The listing builds one solid part. Answer for the finished solid, in the listing's coordinates (mm). A direction names the side the tool comes from. Coordinates: 2 decimals unless noted, no trailing zeros. Order: outer loops, then holes, each group sorted by start corner. A loop starts at its lowest first (then second) coordinate and runs counter-clockwise, first axis right, second up.
from build123d import *

# Parameters (mm, degrees)
F0_R     = 47.826909
F0_R_2   = 27.35277
F1_DEPTH = 12.5
F2_R     = 35.491808
F2_R_2   = 27.557279
F3_DEPTH = 25
F4_R     = 47.701189
F4_R_2   = 35.254813
F5_DEPTH = 12.5
F6_R     = 48.078981
F6_R_2   = 35.711938
F7_DEPTH = 25
F8_R     = 47.890456
F8_R_2   = 35.598206
F9_DEPTH = 25


with BuildPart() as f1:
    # F0 (on Top) → F1 (new body, symmetric)
    with BuildSketch(Plane.XY):
        Circle(F0_R)
        Circle(F0_R_2, mode=Mode.SUBTRACT)
    extrude(amount=F1_DEPTH, both=True)

    # F2 (on Top) → F3 (join, symmetric)
    with BuildSketch(Plane.XY):
        Circle(F2_R)
        Circle(F2_R_2, mode=Mode.SUBTRACT)
    extrude(amount=F3_DEPTH, both=True)

    # F4 (on Top) → F5 (join, symmetric)
    with BuildSketch(Plane.XY):
        Circle(F4_R)
        Circle(F4_R_2, mode=Mode.SUBTRACT)
    extrude(amount=F5_DEPTH, both=True)

    # F6 (on Top) → F7 (cut)
    with BuildSketch(Plane.XY):
        Circle(F6_R)
        Circle(F6_R_2, mode=Mode.SUBTRACT)
    extrude(amount=-F7_DEPTH, mode=Mode.SUBTRACT)

    # F8 (on Top) → F9 (join)
    with BuildSketch(Plane.XY):
        Circle(F8_R)
        Circle(F8_R_2, mode=Mode.SUBTRACT)
    extrude(amount=F9_DEPTH)


solid = f1.part
1) A tool of negligible diameter and unlimited length cuts with its end or side. For faces 4 (the face through (26.285, 8.277, 18.662)), 5 (the face through (26.285, 8.277, -18.838)), 6 (the face through (0, 36, 25)), from which of +Z, -Z, +X, -X, +Y, -Y can it reach the whole face along a straight path? Write none if from no direction.
2) Determine the mould class of faces 1 (the face through (18.2, -20.9, 25)), 2 (the face through (34.06, 10.73, -6.16)), 3 (the face through (-21.71, -16.64, -0.18)) for opening direction Y: released by +Y, released by -Y, zero draft, split by the parting line, or undercut.
3) Section C-C (z = 4) is taken. Give the vertices of the cut face in (x, y), then the cut area to 3 significant figures.
4) Each of these flat-tipped pins is pushed along its axis until it touches: P1, Ø6, axis at x = -28, z = -7.5, coming from the +Y side; P2, Ø5, axis at x = -30, z = -17, coming from the +Y side; P3, Ø2, axis at x = 29, z = -15.5, coming from the +Y side. Where does it stop, or does it pass through?
5) Consider L1, parallel to Y at x = 0, z = -21.5; L2, parallel to Y at x = 0, z = 7.5; L3, parallel to Z at x = 6.5, y = 40. Determine where each line is inside the solid, lowest interval first.
6) Section D-D (y = -34) is taken. Give the vertices of the cut face in (x, z), then the cut area to 3 significant figures.
Filled sheet:
1. face 4: +Z
1. face 5: -Z
1. face 6: +Z, +X, -X, +Y, -Y
2. face 1: zero draft
2. face 2: split by the parting line
2. face 3: undercut
3. outline: circle Ø95.78 at (0, 0); hole circle Ø54.71 at (0, 0)
3. area: 4,850 mm2
4. P1: stops at y = 25.5
4. P2: stops at y = 22.44
4. P3: stops at y = 21.81
5. L1: y = -35.49 to -27.56, 27.56 to 35.49
5. L2: y = -47.89 to -27.35, 27.35 to 47.89
5. L3: z = 0 to 25
6. outline: (-33.73, 0) - (-10.92, 0) - (-10.92, -12.5) - (-10.18, -12.5) - (-10.18, -25) - (10.18, -25) - (10.18, -12.5) - (10.92, -12.5) - (10.92, 0) - (33.73, 0) - (33.73, 25) - (10.55, 25) - (10.55, 12.5) - (10.18, 12.5) - (10.18, 25) - (-10.18, 25) - (-10.18, 12.5) - (-10.55, 12.5) - (-10.55, 25) - (-33.73, 25) - close
6. area: 2,200 mm2
